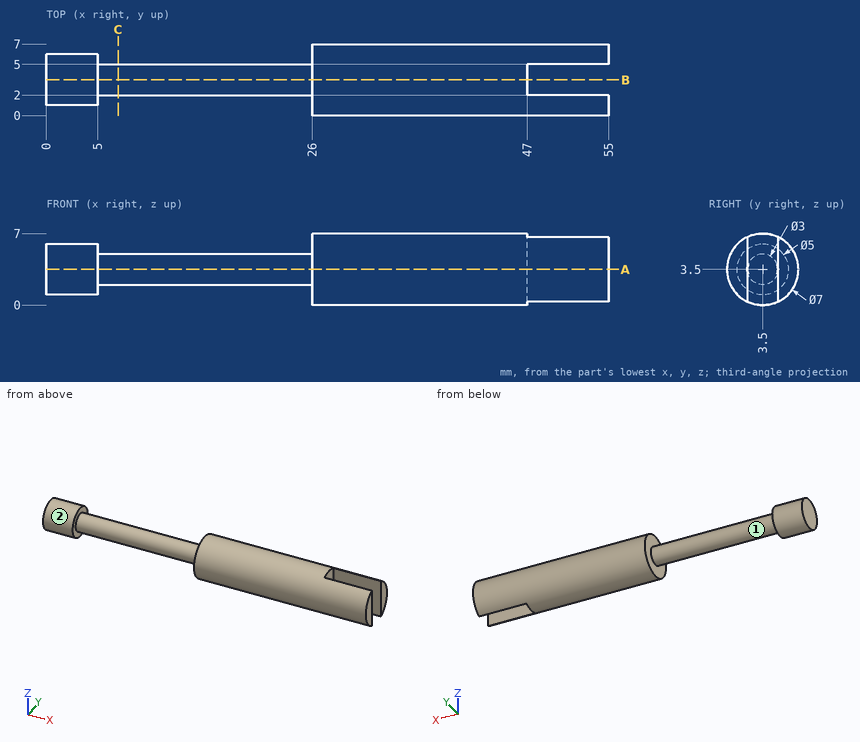
Can you work these out from the drawing? Everything is in mm from the part's minimum corner. Round coordinates to 2 decimals unless told otherwise and drop trailing zeros. Loops run counter-clockwise (first coordinate to the right, second up) from the corner with the lowest first, then second, coordinate; pieces in that order, holes last. Notation, with made-up numbers: (31, 37) - (58, 37) arc R25 cw to (58, 62) - close; hole circle Ø3 at (77, 83.25). An arc over 180 degrees is marked (long way). Answer in a Markdown table with one row per item. Add a question column.
Q1. I want a section at A-A on z = 3.5. List the corners of the cut face in (x, y) for me.
Q2. I need wall thicknesses on L1, parallel to X at y = 4.75, z = 2; L2, parallel to X at y = 4, z = 1; L3, parallel to X at y = 6.25, z = 3.25. Which ranges of each line are inside material? Lowest first, please.
Q3. We'd pull the mould along X, two halves only. Please class the marked faces 1 and 2: pulls with the +X half, pulls with the -X half, needs draft (parallel to the pull), parting line crosses it, or undercut.
Q4. I want a section at C-C on x = 7. List the corners of the cut face in (y, z) for me, and give its area (3 significant figures).
Q5. I want a section at B-B on y = 3.5. List the corners of the cut face in (x, z) for me, and give its area (3 significant figures).
Q6. For pin 1 Ø4 at (x, z) = (9.5, 2.5) entering from +Y; pin 2 Ø3.5 at (y, z) = (4, 2.5) entering from +X; pin 3 Ø1 at (y, z) = (3.5, 3.5) entering from +X; pin 4 Ø2 at (x, y) = (9.5, 4.5) entering from -Z, each with a flat end and sliding along its axis, tell me the tip position at first contact or that it passes through.
A:
| question | item | result |
|---|---|---|
| 1 | outline | (0, 1) - (5, 1) - (5, 2) - (26, 2) - (26, 0) - (55, 0) - (55, 2) - (47, 2) - (47, 5) - (55, 5) - (55, 7) - (26, 7) - (26, 5) - (5, 5) - (5, 6) - (0, 6) - close |
| 2 | L1 | 0 to 5, 26 to 47 |
| 2 | L2 | 26 to 47 |
| 2 | L3 | 26 to 55 |
| 3 | face 1 | undercut |
| 3 | face 2 | needs draft |
| 4 | outline | circle Ø3 at (3.5, 3.5) |
| 4 | area | 7.07 mm^2 |
| 5 | outline | (0, 1) - (5, 1) - (5, 2) - (26, 2) - (26, 0) - (47, 0) - (47, 7) - (26, 7) - (26, 5) - (5, 5) - (5, 6) - (0, 6) - close |
| 5 | area | 235 mm^2 |
| 6 | pin 1 | y = 5 |
| 6 | pin 2 | x = 55 |
| 6 | pin 3 | x = 47 |
| 6 | pin 4 | z = 2 |
